Work out the finished part from the listing and answer in its coordinate system (mm). A direction names the side the tool comes from. Give positions to 0.01 mm unless a question says otherwise; leave off trailing zeros. Loops run counter-clockwise (first coordinate to the right, second up) from the corner with the lowest first, then second, coordinate; pieces in that order, holes last. Notation, with made-up numbers: (-35.5, 27.5) - (-15.5, 27.5) arc R30 cw to (-15.5, 51.5) - close; hole circle Ø5 at (85, 11). An arc over 180 degrees is marked (long way). One line per question, with ' | ' between items.
from build123d import *

# Parameters (mm, degrees)
F0_R      = 12.7
F1_DEPTH  = 3.81
F2_R      = 6.35
F3_DEPTH  = 4.445
F4_R      = 9.525
F5_DEPTH  = 2.54
F6_R      = 6.35
F7_DEPTH  = 4.445
F8_R      = 12.7
F9_DEPTH  = 3.81
F10_R     = 2.54
F11_DEPTH = 19.05


# Not quite as in the source:
# - a fillet or chamfer that OpenCascade refuses, or shapes differently, is made with other operations: its cross-section is extruded or revolved along the edge and cut away or added


with BuildPart() as f1:
    # F0 (on Top) → F1 (new body)
    with BuildSketch(Plane.XY):
        Circle(F0_R)
    extrude(amount=F1_DEPTH)

    # F2 (on face) → F3 (join)
    with BuildSketch(Plane.XY.offset(3.81)):
        Circle(F2_R)
    extrude(amount=F3_DEPTH)

    # F4 (on face) → F5 (join)
    with BuildSketch(Plane.XY.offset(8.255)):
        Circle(F4_R)
    extrude(amount=F5_DEPTH)

    # F6 (on face) → F7 (join)
    with BuildSketch(Plane.XY.offset(10.795)):
        Circle(F6_R)
    extrude(amount=F7_DEPTH)

    # F8 (on face) → F9 (join)
    with BuildSketch(Plane.XY.offset(15.24)):
        with Locations((0, -0.5063372408)):
            Circle(F8_R)
    extrude(amount=F9_DEPTH)

    # F10 (on face) → F11 (cut)
    with BuildSketch(Plane.XY.offset(19.05)):
        Circle(F10_R)
    extrude(amount=-F11_DEPTH, mode=Mode.SUBTRACT)

    # F12: chamfer of 5.08 on 1 edges, made by hand

    # F12_s1 → F12_t2 (revolve, cut)
    with BuildSketch(Plane.XZ.offset(0.5063372408)):
        Polygon((12.7, 13.97), (7.62, 19.05), (12.7, 19.05), align=None)
    revolve(axis=Axis((0, -0.5063372408, 19.05), (0, 0, 1)), mode=Mode.SUBTRACT)

    # F13: chamfer of 5.08 on 1 edges, made by hand

    # F13_s1 → F13_t2 (revolve, cut)
    with BuildSketch(Plane.XZ):
        Polygon((7.62, 0), (12.7, 5.08), (12.7, 0), align=None)
    revolve(axis=Axis((0, 0, 0), (0, 0, 1)), mode=Mode.SUBTRACT)


solid = f1.part
1. Find section A-A on x = 0. Write down the section's boundary in (y, z) (3 decimals), then the cut area to 3 significant figures.
Evaluation:
outline: (-11.936, 15.24) - (-6.35, 15.24) - (-6.35, 10.795) - (-9.525, 10.795) - (-9.525, 8.255) - (-6.35, 8.255) - (-6.35, 3.81) - (-11.43, 3.81) - (-7.62, 0) - (-2.54, 0) - (-2.54, 19.05) - (-8.126, 19.05) - close; (2.54, 0) - (7.62, 0) - (11.43, 3.81) - (6.35, 3.81) - (6.35, 8.255) - (9.525, 8.255) - (9.525, 10.795) - (6.35, 10.795) - (6.35, 15.24) - (10.924, 15.24) - (7.114, 19.05) - (2.54, 19.05) - close | area: 210 mm2
2. Consider L1, parallel to Z at x = 6.25, y = 3.25 (3 decimals); L2, parallel to Z at x = -6.5, y = 6 (3 decimals); L3, parallel to Y at x = 0, z = 12.25. Determine where each line is inside the solid, lowest interval first.
Evaluation:
L1: 0 to 3.81, 8.255 to 10.795, 15.24 to 19.05 | L2: 1.226 to 3.81, 8.255 to 10.795, 15.24 to 17.473 | L3: -6.35 to -2.54, 2.54 to 6.35
3. Find section C-C on y = 8.25. State how many separate pieces and enclosed holes the cut face has, then the cut area to 3 significant figures.
Evaluation:
separate pieces: 3 | enclosed holes: 0 | area: 82.1 mm2
4. Find section B-B on z = 5.25. Write down the section's boundary in (x, y), then the cut area to 3 significant figures.
Evaluation:
outline: circle Ø12.7 at (0, 0); hole circle Ø5.08 at (0, 0) | area: 106 mm2
5. Flat-ended cylindrical pins translate along their axes: pin 1 (1 mm diameter, centred on y = 4.5, z = 7.5, fed in from -X); pin 2 (5 mm diameter, centred on x = 3.5, z = 3, fed in from -Y); pin 3 (8 mm diameter, centred on x = 4.5, z = 12, fed in from +Y). Find the tip coordinate at first contact, or state that the pin passes through.
Evaluation:
pin 1: x = -4.93 | pin 2: y = -11.37 | pin 3: y = 10.72
6. Determine the mould class of faces 1 (the cylindrical face through (-1.38, -6.2, 6)), 2 (the cylindrical face through (-0.33, 2.52, 9.66)), 3 (the flat face through (2, -2, 19.05)) for opening direction Z: +Z half, -Z half, draft (parallel to the pull), parting line (faces both ways), or undercut.
Evaluation:
face 1: undercut | face 2: draft | face 3: +Z half
7. Which of the six approach directions +Z, -Z, +X, -X, +Y, -Y give full straight-line access (tool end or side, diameter ignored) to faces 4 (the flat face through (2, -6.2, 8.255)), 5 (the conical face through (-1.023, 7.791, 0.238))?
Evaluation:
face 4: none | face 5: -Z
